Build history of the part. All positions in model axes, mm. A direction names the side the tool comes from. Coordinates: 2 decimals unless noted, no trailing zeros. Write each loop counter-clockwise with the first axis right and the second up, starting at its lowest first coordinate (ties: lowest second). Pieces come first, ordered by that corner, then holes.
```python
from build123d import *

# Parameters (mm, degrees)
F1_DEPTH = 6.35


with BuildPart() as f1:
    # F0 (on Front) → F1 (new body)
    with BuildSketch(Plane.XZ):
        with BuildLine():
            Line((-6.4141074981, 15.9385126175), (-4.2278079722, 16.9990878248))
            ThreePointArc((-4.2278079722, 16.9990878248), (-1.0521718821, 23.6296872525), (4.699, 19.05))
            ThreePointArc((4.699, 19.05), (4.5806844818, 18.0021781266), (4.2316960296, 17.0071221983))
            Line((4.2316960296, 17.0071221983), (6.4238473824, 15.9488473824))
            Line((6.4238473824, 15.9488473824), (9.1930085155, 21.6849947733))
            Line((9.1930085155, 21.6849947733), (11.9621696486, 27.4211421643))
            ThreePointArc((11.9621696486, 27.4211421643), (-0.0243040276, 29.9167503183), (-12.0067070775, 27.4016701215))
            Line((-12.0067070775, 27.4016701215), (-6.4141074981, 15.9385126175))
        make_face()
        with BuildLine():
            Line((-8.6004070241, 14.8779374102), (-6.4141074981, 15.9385126175))
            Line((-6.4141074981, 15.9385126175), (-12.0067070775, 27.4016701215))
            Line((-12.0067070775, 27.4016701215), (-21.6763890996, 9.1963973453))
            Line((-21.6763890996, 9.1963973453), (-15.9391074981, 6.4135126175))
            Line((-15.9391074981, 6.4135126175), (-14.8789637146, 8.5991379737))
            ThreePointArc((-14.8789637146, 8.5991379737), (-16.1509739914, 16.1496557682), (-8.6004070241, 14.8779374102))
        make_face()
        with BuildLine():
            ThreePointArc((-16.9992346746, -4.227879206), (-23.749, -9.2288e-06), (-16.9992512817, 4.2278872613))
            Line((-16.9992512817, 4.2278872613), (-15.9391074981, 6.4135126175))
            Line((-15.9391074981, 6.4135126175), (-21.6763890996, 9.1963973453))
            Line((-21.6763890996, 9.1963973453), (-27.4136707011, 11.9792820732))
            ThreePointArc((-27.4136707011, 11.9792820732), (-29.9167601905, 3.8177e-06), (-27.4136737585, -11.9792750765))
            Line((-27.4136737585, -11.9792750765), (-15.9391074981, -6.4134484614))
            Line((-15.9391074981, -6.4134484614), (-16.9992346746, -4.227879206))
        make_face()
        with BuildLine():
            Line((-9.1970720847, -21.6758947021), (-6.4141074981, -15.9384484614))
            Line((-6.4141074981, -15.9384484614), (-8.6004236303, -14.8778433301))
            ThreePointArc((-8.6004236303, -14.8778433301), (-16.1509809173, -16.1495205298), (-14.8789803216, -8.5990177168))
            Line((-14.8789803216, -8.5990177168), (-15.9391074981, -6.4134484614))
            Line((-15.9391074981, -6.4134484614), (-27.4136737585, -11.9792750765))
            Line((-27.4136737585, -11.9792750765), (-9.1970720847, -21.6758947021))
        make_face()
        with BuildLine():
            Line((6.4341816168, -15.9384484614), (4.2303024615, -17.0042380186))
            ThreePointArc((4.2303024615, -17.0042380186), (4.5803270771, -18.0006169113), (4.699, -19.05))
            ThreePointArc((4.699, -19.05), (-1.0521904227, -23.6296829928), (-4.227791366, -16.9990535926))
            Line((-4.227791366, -16.9990535926), (-6.4141074981, -15.9384484614))
            Line((-6.4141074981, -15.9384484614), (-9.1970720847, -21.6758947021))
            Line((-9.1970720847, -21.6758947021), (-11.9800366713, -27.4133409429))
            ThreePointArc((-11.9800366713, -27.4133409429), (0.0235983496, -29.9167508833), (12.0232690531, -27.3944071221))
            Line((12.0232690531, -27.3944071221), (6.4341816168, -15.9384484614))
        make_face()
        with BuildLine():
            Line((21.6946431052, -9.1775261509), (15.9591816168, -6.4134484614))
            Line((15.9591816168, -6.4134484614), (14.9083960431, -8.5938286342))
            ThreePointArc((14.9083960431, -8.5938286342), (16.8474784098, -10.3274483008), (17.5673632335, -12.8268969228))
            ThreePointArc((17.5673632335, -12.8268969228), (13.9177463222, -17.4072239999), (8.638060772, -14.8726589042))
            Line((8.638060772, -14.8726589042), (6.4341816168, -15.9384484614))
            Line((6.4341816168, -15.9384484614), (12.0232690531, -27.3944071221))
            Line((12.0232690531, -27.3944071221), (21.6946431052, -9.1775261509))
        make_face()
        with BuildLine():
            Line((15.9488473824, 6.4238473824), (17.0071221983, 4.2316960296))
            ThreePointArc((17.0071221983, 4.2316960296), (21.5481111074, 3.9799550117), (23.749, 0))
            ThreePointArc((23.749, 0), (21.549448622, -3.9791151763), (17.0099671904, -4.2330682886))
            Line((17.0099671904, -4.2330682886), (15.9591816168, -6.4134484614))
            Line((15.9591816168, -6.4134484614), (21.6946431052, -9.1775261509))
            Line((21.6946431052, -9.1775261509), (27.4301045936, -11.9416038403))
            ThreePointArc((27.4301045936, -11.9416038403), (29.9167580877, 0.0112169248), (27.4211421643, 11.9621696486))
            Line((27.4211421643, 11.9621696486), (15.9488473824, 6.4238473824))
        make_face()
        with BuildLine():
            Line((14.8905725665, 8.6159987352), (15.9488473824, 6.4238473824))
            Line((15.9488473824, 6.4238473824), (27.4211421643, 11.9621696486))
            Line((27.4211421643, 11.9621696486), (9.1930085155, 21.6849947733))
            Line((9.1930085155, 21.6849947733), (6.4238473824, 15.9488473824))
            Line((6.4238473824, 15.9488473824), (8.6159987352, 14.8905725665))
            ThreePointArc((8.6159987352, 14.8905725665), (13.8955166382, 17.4283792466), (17.5466947648, 12.8476947648))
            ThreePointArc((17.5466947648, 12.8476947648), (16.8276497765, 10.3495836574), (14.8905725665, 8.6159987352))
        make_face()
        with BuildLine():
            ThreePointArc((-11.0744, 0), (-7.8307833376, 7.8307833376), (0, 11.0744))
            Line((0, 11.0744), (0, 14.351))
            ThreePointArc((0, 14.351), (-2.4943300392, 15.0676742153), (-4.2278079722, 16.9990878248))
            Line((-4.2278079722, 16.9990878248), (-6.4141074981, 15.9385126175))
            Line((-6.4141074981, 15.9385126175), (-8.6004070241, 14.8779374102))
            ThreePointArc((-8.6004070241, 14.8779374102), (-8.2485277438, 13.879197117), (-8.1292149963, 12.827025235))
            ThreePointArc((-8.1292149963, 12.827025235), (-10.3338079753, 8.8447476689), (-14.8789637146, 8.5991379737))
            Line((-14.8789637146, 8.5991379737), (-15.9391074981, 6.4135126175))
            Line((-15.9391074981, 6.4135126175), (-16.9992512817, 4.2278872613))
            ThreePointArc((-16.9992512817, 4.2278872613), (-15.0677224339, 2.494407021), (-14.351, 0))
            Line((-14.351, 0), (-11.0744, 0))
        make_face()
        with BuildLine():
            Line((0, -14.351), (0, -11.0744))
            ThreePointArc((0, -11.0744), (-7.8307833376, -7.8307833376), (-11.0744, 0))
            Line((-11.0744, 0), (-14.351, 0))
            ThreePointArc((-14.351, 0), (-15.0677175349, -2.4943991998), (-16.9992346746, -4.227879206))
            Line((-16.9992346746, -4.227879206), (-15.9391074981, -6.4134484614))
            Line((-15.9391074981, -6.4134484614), (-14.8789803216, -8.5990177168))
            ThreePointArc((-14.8789803216, -8.5990177168), (-10.3338157965, -8.8446144577), (-8.1292149963, -12.8268969228))
            ThreePointArc((-8.1292149963, -12.8268969228), (-8.2485320035, -13.8790873455), (-8.6004236303, -14.8778433301))
            Line((-8.6004236303, -14.8778433301), (-6.4141074981, -15.9384484614))
            Line((-6.4141074981, -15.9384484614), (-4.227791366, -16.9990535926))
            ThreePointArc((-4.227791366, -16.9990535926), (-2.4943139169, -15.0676641171), (0, -14.351))
        make_face()
        with BuildLine():
            Line((14.351, 0), (11.0744, 0))
            ThreePointArc((11.0744, 0), (7.8307833376, -7.8307833376), (0, -11.0744))
            Line((0, -11.0744), (0, -14.351))
            ThreePointArc((0, -14.351), (2.4967544382, -15.0691937657), (4.2303024615, -17.0042380186))
            Line((4.2303024615, -17.0042380186), (6.4341816168, -15.9384484614))
            Line((6.4341816168, -15.9384484614), (8.638060772, -14.8726589042))
            ThreePointArc((8.638060772, -14.8726589042), (9.5434199744, -9.506452175), (14.9083960431, -8.5938286342))
            Line((14.9083960431, -8.5938286342), (15.9591816168, -6.4134484614))
            Line((15.9591816168, -6.4134484614), (17.0099671904, -4.2330682886))
            ThreePointArc((17.0099671904, -4.2330682886), (15.0708848237, -2.499448622), (14.351, 0))
        make_face()
        with BuildLine():
            ThreePointArc((0, 11.0744), (7.8307833376, 7.8307833376), (11.0744, 0))
            Line((11.0744, 0), (14.351, 0))
            ThreePointArc((14.351, 0), (15.0700449883, 2.4981111074), (17.0071221983, 4.2316960296))
            Line((17.0071221983, 4.2316960296), (15.9488473824, 6.4238473824))
            Line((15.9488473824, 6.4238473824), (14.8905725665, 8.6159987352))
            ThreePointArc((14.8905725665, 8.6159987352), (9.525, 9.525), (8.6159987352, 14.8905725665))
            Line((8.6159987352, 14.8905725665), (6.4238473824, 15.9488473824))
            Line((6.4238473824, 15.9488473824), (4.2316960296, 17.0071221983))
            ThreePointArc((4.2316960296, 17.0071221983), (2.4981111074, 15.0700449883), (0, 14.351))
            Line((0, 14.351), (0, 11.0744))
        make_face()
    extrude(amount=F1_DEPTH)


solid = f1.part
```
1. Saw through at D-D on y = -5.5. State how many separate pieces and enclosed holes the cut face has, plus the area to 3 significant figures.
Computed values:
separate pieces: 1
enclosed holes: 9
area: 1,490 mm2
2. Saw through at A-A on x = 16. List the corners of the cut face in (y, z), plus the area to 3 significant figures.
Computed values:
outline: (-6.35, -19.9) - (0, -19.9) - (0, -16.33) - (-6.35, -16.33) - close; (-6.35, -9.32) - (0, -9.32) - (0, -3.57) - (-6.35, -3.57) - close; (-6.35, 3.57) - (0, 3.57) - (0, 9.36) - (-6.35, 9.36) - close; (-6.35, 16.33) - (0, 16.33) - (0, 18.05) - (-6.35, 18.05) - close
area: 107 mm2
3. Probe line 1 along Z through (x, y) = (0.5, -0.5); line 2 along X through (y, z) = (-0.75, 13); line 3 along X through (y, z) = (-0.75, -15.5). List the from-to ranges inside material, lowest first.
Computed values:
line 1: z = -29.91 to -23.72, -14.38 to -11.06, 11.06 to 14.38, 23.72 to 29.91
line 2: x = -19.66 to -17.52, -8.13 to 8.15, 17.54 to 25.48
line 3: x = -20.8 to -16.69, -8.96 to -3.08, 3.08 to 9, 16.73 to 18.34
4. Saw through at B-B on x = -10. List the corners of the cut face in (y, z), plus the area to 3 significant figures.
Computed values:
outline: (-6.35, -28.2) - (0, -28.2) - (0, -23.33) - (-6.35, -23.33) - close; (-6.35, -21.25) - (0, -21.25) - (0, -16.58) - (-6.35, -16.58) - close; (-6.35, -9.07) - (0, -9.07) - (0, -4.76) - (-6.35, -4.76) - close; (-6.35, 4.76) - (0, 4.76) - (0, 9.07) - (-6.35, 9.07) - close; (-6.35, 16.58) - (0, 16.58) - (0, 28.2) - (-6.35, 28.2) - close
area: 189 mm2
5. Mould opens along X. For faces 3 (the face through (-10.569, -3.131, -24.504)), 4 (the face through (24.52, -3.13, -10.54)), 5 (the face through (-24.505, -3.131, 10.568)), 6 (the face through (-0.149, -3.131, -29.916)) say: +X half, -X half, draft (parallel to the pull), parting line (faces both ways), or undercut.
Computed values:
face 3: -X half
face 4: undercut
face 5: undercut
face 6: parting line
6. Flat gauge pins, fed straight in: pin 1 (2 mm diameter, centred on x = 8, z = -16.5, fed in from +Y); pin 2 (1 mm diameter, centred on y = -2.5, z = -19, fed in from +X); pin 3 (3 mm diameter, centred on x = 6.5, y = -3.5, fed in from +Z). Where does each tip first touch, or does it go through?
Computed values:
pin 1: stops at y = 0
pin 2: stops at x = 16.75
pin 3: stops at z = 29.5
7. Saw through at C-C on x = -19.05. List the corners of the cut face in (y, z), plus the area to 3 significant figures.
Computed values:
outline: (-6.35, -16.43) - (0, -16.43) - (0, -4.7) - (-6.35, -4.7) - close; (-6.35, 4.7) - (0, 4.7) - (0, 14.14) - (-6.35, 14.14) - close
area: 134 mm2
8. 3-axis set-ups, long thin cutter, end or side, ignore diameter. For faces 1 (the face through (13, -6.35, 0)), 2 (the face through (10.558, -3.131, 24.513)): which of +Z, -Z, +X, -X, +Y, -Y reach the whole face in a straight line?
Computed values:
face 1: +Z, -Z, +X, -X, -Y
face 2: +X, +Y, -Y
